Can you work these out from the model? Positions are in its coordinate system, mm. A direction names the side the tool comes from. Round coordinates to 2 decimals unless told otherwise and drop trailing zeros. Order: outer loops, then holes, each group sorted by start corner. A loop starts at its lowest first (then second) coordinate and runs counter-clockwise, first axis right, second up.
Q1. If we section it at C-C (x = 19.05): Please give me the cut outline in (y, z).
Q2. Will this pin go through, and if not, where does the flat tip stop? P1, Ø6, axis at x = 31, z = 9.5, coming from the -Y side.
Q3. If we section it at D-D (x = 13.5): Please give me the cut outline in (y, z), plus the area to 3 significant figures.
Q4. If we section it at A-A (z = 17): Please give me the cut outline in (x, y).
Q5. For faces 1 (the face through (12.7, -13, 19)), 2 (the face through (38.1, -13, 13)), 3 (the face through (2.54, -14, 13)), which set-ups out of +Z, -Z, +X, -X, +Y, -Y let a thin tool reach every point of the face, with its end or its side?
Q6. If I drill on line 1 (X direction, y = -9, z = 13.75); line 2 (Z direction, x = 34, y = -15.5); line 3 (X direction, y = -22.25, z = 5.75), over which ranges is the centre line in solid material (lowest first)?
Q7. We'd pull the mould along X, two halves only. Please class faces 4 (the face through (19, -13, 0)), 5 (the face through (6, -14, 22.86)), 6 (the face through (0, -13, 13)): pulls with the +X half, pulls with the -X half, needs draft (parallel to the pull), parting line crosses it, or undercut.
Q8. If we section it at B-B (y = -21.5): Please give me the cut outline in (x, z), plus the area to 3 significant figures.
from build123d import *

# Parameters (mm, degrees)
F0_W     = 38.1
F0_H     = 25.4
F0_R     = 6.35
F1_DEPTH = 25.4
F2_W     = 12.7
F2_H     = 25.4
F3_DEPTH = 12.7
F4_T     = -2.54


with BuildPart() as f1:
    # F0 (on Front) → F1 (new body)
    with BuildSketch(Plane.XZ):
        with Locations((19.05, 12.7)):
            Rectangle(F0_W, F0_H)
        with Locations((19.05, 12.7)):
            Circle(F0_R, mode=Mode.SUBTRACT)
    extrude(amount=F1_DEPTH)

    # F2 (on face) → F3 (cut)
    with BuildSketch(Plane.XY.offset(25.4)):
        with Locations((19.05, -12.7)):
            Rectangle(F2_W, F2_H)
    extrude(amount=-F3_DEPTH, mode=Mode.SUBTRACT)

    # F4
    f4_openings = [f1.faces().sort_by_distance(p)[0] for p in [
        (6.35, -25.4, 24.942095),
    ]]
    offset(amount=F4_T, openings=f4_openings)


solid = f1.part
Solution:
1. outline: (-25.4, 0) - (0, 0) - (0, 6.35) - (-25.4, 6.35) - (-25.4, 3.81) - (-2.54, 3.81) - (-2.54, 2.54) - (-25.4, 2.54) - close
2. P1: stops at y = -2.54
3. outline: (-25.4, 0) - (0, 0) - (0, 9.61) - (-25.4, 9.61) - (-25.4, 5.76) - (-2.54, 5.76) - (-2.54, 2.54) - (-25.4, 2.54) - close
3. area: 171 mm2
4. outline: (0, -25.4) - (2.54, -25.4) - (2.54, -2.54) - (10.16, -2.54) - (10.16, -25.4) - (12.7, -25.4) - (12.7, 0) - (0, 0) - close; (25.4, -25.4) - (27.94, -25.4) - (27.94, -2.54) - (35.56, -2.54) - (35.56, -25.4) - (38.1, -25.4) - (38.1, 0) - (25.4, 0) - close
5. face 1: +Z, +Y, -Y
5. face 2: +Z, -Z, +X, +Y, -Y
5. face 3: -Y
6. line 1: x = 0 to 2.54, 10.16 to 12.7, 25.4 to 27.94, 35.56 to 38.1
6. line 2: z = 0 to 2.54, 22.86 to 25.4
6. line 3: x = 0 to 2.54, 13.51 to 24.59, 35.56 to 38.1
7. face 4: needs draft
7. face 5: undercut
7. face 6: pulls with the -X half
8. outline: (0, 0) - (38.1, 0) - (38.1, 25.4) - (25.4, 25.4) - (25.4, 12.7) arc R6.35 cw to (12.7, 12.7) - (12.7, 25.4) - (0, 25.4) - close; hole (2.54, 2.54) - (35.56, 2.54) - (35.56, 22.86) - (27.94, 22.86) - (27.94, 12.7) arc R8.89 cw to (10.16, 12.7) - (10.16, 22.86) - (2.54, 22.86) - close
8. area: 377 mm2
